Source: CAD feature listing. Evaluate the final solid. Frame: model axes, mm. A direction names the side the tool comes from. Coordinates: 2 decimals unless noted, no trailing zeros. Write each loop counter-clockwise with the first axis right and the second up, starting at its lowest first coordinate (ties: lowest second). Pieces come first, ordered by that corner, then holes. Notation, with made-up numbers: (76, 21) -> (98, 21) arc R36 cw to (98, 60) -> close; hole circle Ø7 at (40, 76). An arc over 180 degrees is marked (long way). One line per item, written item: value. Start each with the question number.
1. Section query B-B, the plane z = 0. Output: boundary loops of the cut face in (x, y).
2. Section query A-A, the plane x = 0. Output: boundary loops of the cut face in (y, z).
3. First-contact query: P1, Ø1.2, axis at x = -0.5, z = -0.5, coming from the -Y side; P2, Ø5, axis at x = -3.5, y = 27.5, coming from the -Z side; P3, Ø1.2, axis at x = 0, z = -1, coming from the +Y side. Flat tips, straight axial feed; report the tip coordinate or a pass-through.
4. Access query for faces 4 (the flat face through (2, 0, 2)), 5 (the cylindrical face through (1.26, 103.92, -1.64)), 6 (the flat face through (0, 12, 0)). Directions: +Z, -Z, +X, -X, +Y, -Y. A direction counts if a zero-diameter tool reaches every point of the face in a straight line with its end or side. Return the directions, or none.
5. Section query C-C, the plane y = 48. Output: boundary loops of the cut face in (x, z), and give its area (3 significant figures).
6. Line query: line 1 (X direction, y = 100.5, z = 0); line 2 (Z direction, x = -3, y = 39.5). Output: solid intervals per line, ascending.
7. Mould query, pull axis Z, two halves, no side actions, for faces 1 (the cylindrical face through (-1.08, 54.24, -4.88)), 2 (the flat face through (2, 110, 2)), 3 (the cylindrical face through (1.26, 6.08, 1.64)). Classes: released by +Z, released by -Z, zero draft, split by the parting line, or undercut.
Autodesk Inventor part; units mm, degrees
ref_plane "YZ Plane" through (0, 0, 0) normal (1, 0, 0) x (0, 1, 0)
ref_plane "XZ Plane" through (0, 0, 0) normal (0, 1, 0) x (-1, 0, 0)
ref_plane "XY Plane" through (0, 0, 0) normal (0, 0, 1) x (1, 0, 0)
sketch "Sketch1" plane through (0, 0, 0) normal (0, 0, 1) x (1, 0, 0)
  line L0 (0, 0) -> (0, 110)
  line L1 (0, 110) -> (5, 110)
  line L2 (5, 110) -> (5, 0)
  line L3 (5, 0) -> (0, 0)
  dimension "d0" = 110
  dimension "d1" = 10
revolve "Revolution1" add sketch "Sketch1" angle 360 about axis through (0, 0, 0) along (0, 1, 0)
fillet "Fillet1" radius 1 2 edges at (-5, 0, 0) (-5, 110, 0)
sketch "Sketch2" plane through (0, 110, 0) normal (0, 1, 0) x (1, 0, 0)
  circle A0 centre (0, 0) radius 5
hole "Hole1" at (0, 110, 0) direction (0, -1, 0) diameter 4.134 depth 12
sketch "Sketch3" plane through (0, 0, 0) normal (0, -1, 0) x (1, 0, 0)
  circle A0 centre (0, 0) radius 5
hole "Hole2" at (0, 0, 0) direction (0, 1, 0) diameter 4.134 depth 12
properties part number "121"
Computed values:
1. outline: (-5, 1) arc R1 ccw to (-4, 0) -> (-2.07, 0) -> (-2.07, 12) -> (2.07, 12) -> (2.07, 0) -> (4, 0) arc R1 ccw to (5, 1) -> (5, 109) arc R1 ccw to (4, 110) -> (2.07, 110) -> (2.07, 98) -> (-2.07, 98) -> (-2.07, 110) -> (-4, 110) arc R1 ccw to (-5, 109) -> close
2. outline: (0, -4) arc R1 ccw to (1, -5) -> (109, -5) arc R1 ccw to (110, -4) -> (110, -2.07) -> (98, -2.07) -> (98, 2.07) -> (110, 2.07) -> (110, 4) arc R1 ccw to (109, 5) -> (1, 5) arc R1 ccw to (0, 4) -> (0, 2.07) -> (12, 2.07) -> (12, -2.07) -> (0, -2.07) -> close
3. P1: stops at y = 12
3. P2: stops at z = -4.9
3. P3: stops at y = 98
4. face 4: +Z, -Z, +X, -X, -Y
4. face 5: +Y
4. face 6: -Y
5. outline: circle Ø10 at (0, 0)
5. area: 78.5 mm²
6. line 1: x = -5 to -2.07, 2.07 to 5
6. line 2: z = -4 to 4
7. face 1: split by the parting line
7. face 2: zero draft
7. face 3: undercut
